Geometry: see drawing. Coordinates: mm, zero at the bounding-box minimum. A direction names the side the tool comes from. Coordinates: 2 decimals unless noted, no trailing zeros. Loops run counter-clockwise (first coordinate to the right, second up) from the corner with the lowest first, then second, coordinate; pieces in that order, holes last. Notation, with made-up numbers: (73.25, -36.5) -> (131.25, -36.5) arc R11 ccw to (131.25, -24.5) -> close; hole circle Ø5 at (79.5, 17.5). An arc over 180 degrees is marked (long way). One line per question, with ' | ' between items. Start each with the question number.
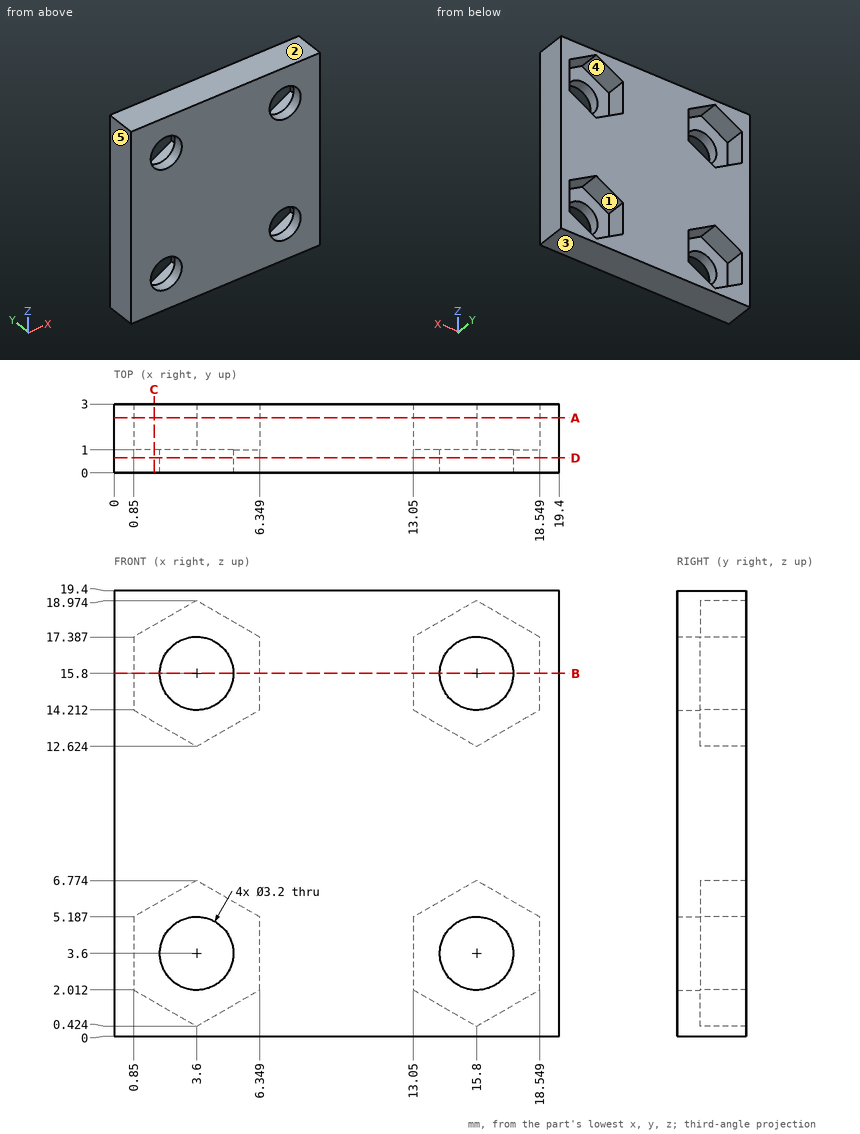
(1) Ray query, L1, parallel to X at y = 0.5, z = 15.8; L2, parallel to X at y = 1.65, z = 2.5. Return the intervals inside material, ascending.
(2) Contact query for flat-ended pins moving along their axis: pin 1 Ø10 at (x, z) = (14.5, 4.5) entering from -Y; pin 2 Ø1.9 at (x, z) = (3.6, 15.8) entering from +Y. Output: stop coordinate, or through.
(3) Cut plane D-D, the plane y = 0.65. Return the cut outline in (x, z), and give its area (3 significant figures).
(4) Cut plane B-B, the plane z = 15.8. Return the cut outline in (x, y).
(5) Cut plane C-C, the plane x = 1.75. Return the cut outline in (y, z).
(6) Draft query along Z for the marked faces 1, 2 and 3. Return one class per face: pulls with the +Z half, pulls with the -Z half, needs draft (parallel to the pull), parting line crosses it, or undercut.
(7) Access query for the marked faces 4 and 5. Directions: +Z, -Z, +X, -X, +Y, -Y. A direction counts if a zero-diameter tool reaches every point of the face in a straight line with its end or side. Return the directions, or none.
(8) Cut plane A-A, the plane y = 2.4. State how many separate pieces and enclosed holes the cut face has.
Here are the results:
1) L1: x = 0 to 2, 5.2 to 14.2, 17.4 to 19.4 | L2: x = 0 to 0.85, 6.35 to 13.05, 18.55 to 19.4
2) pin 1: stops at y = 0 | pin 2: passes through
3) outline: (0, 0) -> (19.4, 0) -> (19.4, 19.4) -> (0, 19.4) -> close; hole circle Ø3.2 at (3.6, 3.6); hole circle Ø3.2 at (3.6, 15.8); hole circle Ø3.2 at (15.8, 3.6); hole circle Ø3.2 at (15.8, 15.8) | area: 344 mm2
4) outline: (0, 0) -> (2, 0) -> (2, 1) -> (0.85, 1) -> (0.85, 3) -> (0, 3) -> close; (5.2, 0) -> (14.2, 0) -> (14.2, 1) -> (13.05, 1) -> (13.05, 3) -> (6.35, 3) -> (6.35, 1) -> (5.2, 1) -> close; (17.4, 0) -> (19.4, 0) -> (19.4, 3) -> (18.55, 3) -> (18.55, 1) -> (17.4, 1) -> close
5) outline: (0, 0) -> (3, 0) -> (3, 1.49) -> (1, 1.49) -> (1, 5.71) -> (3, 5.71) -> (3, 13.69) -> (1, 13.69) -> (1, 17.91) -> (3, 17.91) -> (3, 19.4) -> (0, 19.4) -> close
6) face 1: undercut | face 2: pulls with the +Z half | face 3: pulls with the -Z half
7) face 4: +Y | face 5: +Z, -Z, -X, +Y, -Y
8) separate pieces: 1 | enclosed holes: 4
